from build123d import *

# Parameters (mm, degrees)
BOSS_EXTRUDE1_DEPTH            = 12.75
BOSS_EXTRUDE1_DEPTH_BACK       = 12.75
SKETCH1_R                      = 4.5
CUT_EXTRUDE1_DEPTH             = 4
CUT_EXTRUDE3_REACH             = 16.25
SKETCH4_R                      = 1.6
CUT_EXTRUDE3_DIRECTION_2_REACH = 16.25


with BuildPart() as part:
    # Sketch1 → Boss-Extrude1 (new, two sides: drawn at the far end of the back side and taken through both)
    with BuildSketch(Plane(origin=(0, 0, 0), x_dir=(0, 0, -1), z_dir=(1, 0, 0)).offset(-BOSS_EXTRUDE1_DEPTH_BACK)):
        with Locations(Location((0, 0, 0), (0, 0, 180))):
            Circle(SKETCH1_R)
    extrude(amount=BOSS_EXTRUDE1_DEPTH + BOSS_EXTRUDE1_DEPTH_BACK)

    # Sketch2 → Cut-Extrude1 (cut)
    with BuildSketch(Plane.ZY.offset(12.75)):
        Polygon((3.157465818, -0.337257977), (1.870806885, 2.565816621), (-1.286658933, 2.903074598), (-3.157465818, 0.337257977), (-1.870806885, -2.565816621), (1.286658933, -2.903074598), align=None)
    cut_extrude1 = extrude(amount=-CUT_EXTRUDE1_DEPTH, mode=Mode.SUBTRACT)

    # Mirror1: Cut-Extrude1 across plane
    add(cut_extrude1.mirror(Plane(origin=(0, 0, 0), x_dir=(0, 0, 1), z_dir=(1, 0, 0))), mode=Mode.SUBTRACT)

    # Cut-Extrude3: up to this face of the body (flat: up to its plane)
    cut_extrude3_end = Plane(part.part.faces().sort_by_distance((-8.75, 0, 0))[0])
    # Sketch4 → Cut-Extrude3 (cut, up to the picked face)
    with BuildSketch(Plane(origin=(0, 0, 0), x_dir=(0, 0, -1), z_dir=(1, 0, 0)), mode=Mode.PRIVATE) as cut_extrude3_sk1:
        Circle(SKETCH4_R)
    cut_extrude3_tool1 = split(extrude(cut_extrude3_sk1.sketch, amount=-CUT_EXTRUDE3_REACH, mode=Mode.PRIVATE), bisect_by=cut_extrude3_end, keep=Keep.BOTH, mode=Mode.PRIVATE)
    add(cut_extrude3_tool1.solids().sort_by(Axis((0, 0, 0), (-1, 0, 0)))[0], mode=Mode.SUBTRACT)

    # Cut-Extrude3 direction 2: up to this face of the body (flat: up to its plane)
    cut_extrude3_direction_2_end = Plane(part.part.faces().sort_by_distance((8.75, 0, 0))[0])
    # Sketch4 → Cut-Extrude3 direction 2 (cut, up to the picked face)
    with BuildSketch(Plane(origin=(0, 0, 0), x_dir=(0, 0, -1), z_dir=(1, 0, 0)), mode=Mode.PRIVATE) as cut_extrude3_direction_2_sk1:
        Circle(SKETCH4_R)
    cut_extrude3_direction_2_tool1 = split(extrude(cut_extrude3_direction_2_sk1.sketch, amount=CUT_EXTRUDE3_DIRECTION_2_REACH, mode=Mode.PRIVATE), bisect_by=cut_extrude3_direction_2_end, keep=Keep.BOTH, mode=Mode.PRIVATE)
    add(cut_extrude3_direction_2_tool1.solids().sort_by(Axis((0, 0, 0), (1, 0, 0)))[0], mode=Mode.SUBTRACT)


solid = part.part
The model under review builds one solid part; all positions refer to its coordinate system, in mm. A direction names the side the tool comes from. Give positions to 0.01 mm unless a question says otherwise; leave off trailing zeros. Loops run counter-clockwise (first coordinate to the right, second up) from the corner with the lowest first, then second, coordinate; pieces in that order, holes last. Notation, with made-up numbers: (87, 68.25) -> (115, 68.25) arc R23 cw to (115, 105.25) -> close; hole circle Ø4 at (21.5, 20). An arc over 180 degrees is marked (long way). Write each question's results on one line, items separated by ' | '.
1) Take a section at D-D, the plane x = -2.75. Give the boundary of the cut face in (y, z), plus the area to 3 significant figures.
Conclusion:
outline: circle Ø9 at (0, 0); hole circle Ø3.2 at (0, 0) | area: 55.6 mm^2
2) Tool access review of faces 5 (the face through (-10.778, 2.732, 0.314)), 6 (the face through (-12.75, 3, 0)), 7 (the face through (10.778, -1.094, -2.523)): name each direction out of +Z, -Z, +X, -X, +Y, -Y from which nothing blocks a thin tool from reaching the whole face with its end or side.
Conclusion:
face 5: -X | face 6: +Z, -Z, -X, +Y, -Y | face 7: +X
3) Take a section at B-B, the plane z = 0. Give the boundary of the cut face in (x, y), plus the area to 3 significant figures.
Conclusion:
outline: (-12.75, -4.5) -> (12.75, -4.5) -> (12.75, -2.77) -> (8.75, -2.77) -> (8.75, -1.6) -> (-8.75, -1.6) -> (-8.75, -2.77) -> (-12.75, -2.77) -> close; (-12.75, 2.77) -> (-8.75, 2.77) -> (-8.75, 1.6) -> (8.75, 1.6) -> (8.75, 2.77) -> (12.75, 2.77) -> (12.75, 4.5) -> (-12.75, 4.5) -> close | area: 129 mm^2
4) Take a section at C-C, the plane z = -2.25. Give the boundary of the cut face in (x, y), plus the area to 3 significant figures.
Conclusion:
outline: (-12.75, -3.9) -> (12.75, -3.9) -> (12.75, -1.71) -> (8.75, -1.71) -> (8.75, 1.58) -> (12.75, 1.58) -> (12.75, 3.9) -> (-12.75, 3.9) -> (-12.75, 1.58) -> (-8.75, 1.58) -> (-8.75, -1.71) -> (-12.75, -1.71) -> close | area: 172 mm^2
5) Insertion check: pin 1 Ø4 at (x, z) = (-4.5, 3) entering from -Y; pin 2 Ø4.5 at (y, z) = (0, -0.5) entering from -X; pin 3 Ø1.5 at (x, z) = (-8, 1.5) entering from +Y. Each pin has a flat end and moves straight along its axis. Give the tip position at first contact, or say it passes through.
Conclusion:
pin 1: stops at y = -4.39 | pin 2: stops at x = -8.75 | pin 3: stops at y = 4.44
6) For line 1 along X through (y, z) = (1.75, -1); line 2 along Y through (x, z) = (4.5, 0); line 3 along Z through (x, y) = (1, -0.5), list the stretches that pass through material, from the lowest coordinate up. Write a range as from..to.
Conclusion:
line 1: x = -8.75..8.75 | line 2: y = -4.5..-1.6, 1.6..4.5 | line 3: z = -4.47..-1.52, 1.52..4.47
7) Take a section at A-A, the plane y = 0. Give the boundary of the cut face in (x, z).
Conclusion:
outline: (-12.75, -4.5) -> (12.75, -4.5) -> (12.75, -3.01) -> (8.75, -3.01) -> (8.75, -1.6) -> (-8.75, -1.6) -> (-8.75, -3.01) -> (-12.75, -3.01) -> close; (-12.75, 3.01) -> (-8.75, 3.01) -> (-8.75, 1.6) -> (8.75, 1.6) -> (8.75, 3.01) -> (12.75, 3.01) -> (12.75, 4.5) -> (-12.75, 4.5) -> close
8) Draft analysis for pull direction Z (two halves, no side actions). For faces 1 (the face through (-0.18, -3.04, -3.32)), 2 (the face through (-8.75, -1.2, -1.4)), 3 (the face through (12.75, 3, 0)), 4 (the face through (0.12, -0.97, 1.27)), state which applies: pulls with the +Z half, pulls with the -Z half, needs draft (parallel to the pull), parting line crosses it, or undercut.
Conclusion:
face 1: parting line crosses it | face 2: undercut | face 3: needs draft | face 4: undercut
